Design review of the part shown in the three views and the two pictorial views. Dimensions are in mm from the part's minimum x, y and z. A direction names the side the tool comes from. Coordinates: 2 decimals unless noted, no trailing zeros. Loops run counter-clockwise (first coordinate to the right, second up) from the corner with the lowest first, then second, coordinate; pieces in that order, holes last.
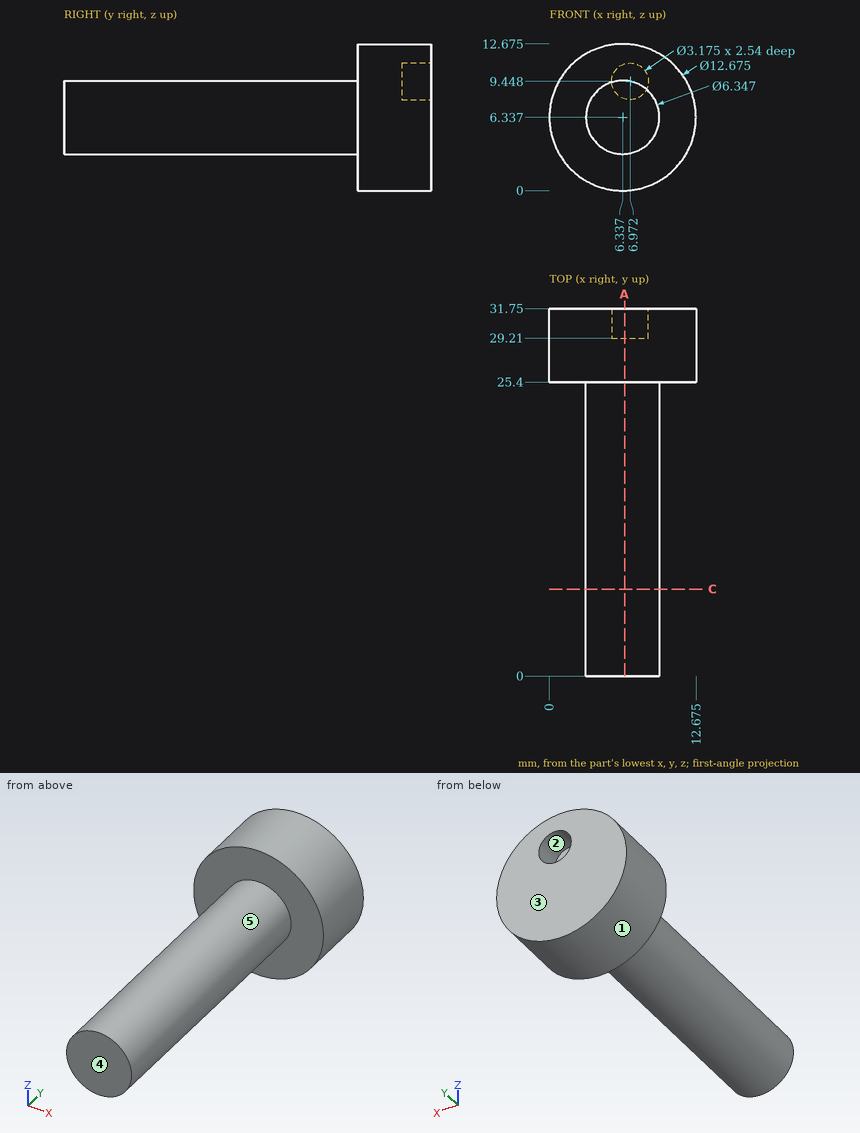
Q1. Wall thickness on probe 1 along Y at (x, z) = (7.75, 12.25); probe 2 along X at (y, z) = (23.5, 6.5); probe 3 along Y at (x, z) = (5.5, 9): over which ranges is each line inside the solid? List them lowest first.
Q2. Consider section A-A (x = 6.5). State the section outline as (y, z) points.
Q3. For pin 1 Ø1.5 at (x, y) = (3.5, 25.5) entering from -Z; pin 2 Ø6 at (x, y) = (11, 15) entering from -Z (1 decimal); pin 3 Ø6 at (x, y) = (8.5, 11) entering from +Z, all flat-tipped, find the tip position at first contact; note any pin that passes through.
Q4. The part is to be moulded in two halves that separate along Z. For the marked faces 1, 2 and 3, say which applies: +Z half, -Z half, draft (parallel to the pull), parting line (faces both ways), or undercut.
Q5. Consider section C-C (y = 7.5). State the section outline as (x, z) points.
Q6. Machinability: for the marked faces 4 and 5, which of the approach directions +Z, -Z, +X, -X, +Y, -Y give a long, thin tool a straight path to every point of the face, cutting with its end or side? Answer none if there is none.
Model answer:
1. probe 1: y = 25.4 to 31.75
1. probe 2: x = 3.17 to 9.51
1. probe 3: y = 0 to 29.21
2. outline: (0, 3.17) - (25.4, 3.17) - (25.4, 0) - (31.75, 0) - (31.75, 7.93) - (29.21, 7.93) - (29.21, 10.96) - (31.75, 10.96) - (31.75, 12.67) - (25.4, 12.67) - (25.4, 9.51) - (0, 9.51) - close
3. pin 1: stops at z = 0.35
3. pin 2: stops at z = 3.6
3. pin 3: stops at z = 9.51
4. face 1: parting line
4. face 2: undercut
4. face 3: draft
5. outline: circle Ø6.35 at (6.34, 6.34)
6. face 4: +Z, -Z, +X, -X, -Y
6. face 5: -Y
